Input: part model. Units: mm. Frame: model coordinates. A direction names the side the tool comes from. Coordinates: 2 decimals unless noted, no trailing zeros. Write each loop counter-clockwise with the first axis right and the second up, starting at its lowest first coordinate (ties: lowest second). Pieces come first, ordered by that corner, then holes. Notation, with made-up numbers: (50.5, 17.25) - (79.5, 17.25) arc R13 cw to (79.5, 39.25) - close; hole circle Ø6 at (43.5, 15). An arc over 180 degrees is marked (long way). Put each result on its own line as item: value. Start each with the question number.
1. Cut plane B-B, the plane z = -44. Return loops of the section in (x, y), and give its area (3 significant figures).
2. Access query for faces 1 (the flat face through (5.151, 45.99, -111.247)), 2 (the cylindrical face through (6.28, 102.887, -89.304)), 3 (the flat face through (5, 58.8, -29.4)), 4 (the flat face through (5, -5, -84.398)), 5 (the flat face through (5, -10.16, -117)). Directions: +Z, -Z, +X, -X, +Y, -Y. A direction counts if a zero-diameter tool reaches every point of the face in a straight line with its end or side. Return the directions, or none.
3. Line query: line 1 (Z direction, x = 5.75, y = 66.5); line 2 (Z direction, x = 9, y = 44); line 3 (Y direction, x = 0.5, z = -44). Output: solid intervals per line, ascending.
4. Cut plane A-A, the plane y = 24.5. Return loops of the section in (x, z), and give its area (3 significant figures).
5. Cut plane C-C, the plane z = -133.5. Return loops of the section in (x, y), and give its area (3 significant figures).
6. Pull-direction query (Y, two-part tool) for faces 6 (the flat face through (2.667, -5, -117)), 7 (the flat face through (5.151, 45.99, -38.753)), 8 (the flat face through (5, -10.16, -75)), 9 (the cylindrical face through (2.576, 103.424, -84.174)); classes: released by +Y, released by -Y, zero draft, split by the parting line, or undercut.
7. Pin query (flat end, axial travel): pin 1 (2.5 mm diameter, centred on x = 6, y = -3, fed in from +Z); pin 2 (4 mm diameter, centred on x = 4, y = -3, fed in from -Z); pin 3 (3 mm diameter, centred on x = 6, y = 27, fed in from +Z); pin 4 (5 mm diameter, centred on y = 36, z = -132, fed in from -X). Return the tip coordinate at first contact, or that it passes through.
Autodesk Inventor part; units mm, degrees
ref_plane "YZ Plane" through (0, 0, 0) normal (1, 0, 0) x (0, 1, 0)
ref_plane "XZ Plane" through (0, 0, 0) normal (0, 1, 0) x (-1, 0, 0)
ref_plane "XY Plane" through (0, 0, 0) normal (0, 0, 1) x (1, 0, 0)
sketch "Sketch1" plane through (0, 0, 0) normal (1, 0, 0) x (0, 1, 0)
  line L0 (150, -75) -> (0, 0)
  line L1 (150, -75) -> (0, -150)
  line L2 (0, -150) -> (0, 0)
  dimension "d0" = 150
  dimension "d1" = 75
extrude "Extrusion1" add sketch "Sketch1" along normal blind 10.16
sketch "Sketch2" plane through (10.16, 0, 0) normal (1, 0, 0) x (0, 0, -1)
  point P0 (0, 0)
fillet "Fillet1" radius 19.05 1 edges at (5.08, 150, -75)
sketch "Sketch3" plane through (10.16, 0, 0) normal (1, 0, 0) x (0, 0, -1)
  arc A0 (92.0388, 115.9223) -> (57.9612, 115.9223) centre (75, 107.4029) ccw
  circle A1 centre (75, 107.4029) radius 15
  circle A2 centre (75, 107.4029) radius 10
  line L0 (75, 122.4029) -> (75, 117.4029)
  line L1 (75, 97.4029) -> (75, 92.4029)
  line L2 (85.6066, 118.0095) -> (82.0711, 114.474)
  line L3 (67.9289, 100.3318) -> (64.3934, 96.7963)
  point P0 (0, 0)
  dimension "d5" = 30
  dimension "d34" = 20
  dimension "d35" = 45
  dimension "d36" = 45
sketch "Sketch4" plane through (10.16, 0, 0) normal (1, 0, 0) x (0, 0, -1)
  line L0 (22.8055, 14.0945) -> (60.9055, 90.2945)
  line L1 (57.9612, 115.9223) -> (0, 0)
  line L2 (22.8055, 14.0945) -> (60.9055, 14.0945)
  line L3 (60.9055, 14.0945) -> (60.9055, 90.2945)
  line L4 (0, 0) -> (150, 0) construction
  line L5 (0, 0) -> (150, 0) construction
  arc A0 (92.0388, 115.9223) -> (57.9612, 115.9223) centre (75, 107.4029) ccw construction
  line L6 (75, 126.4529) -> (75, 0) construction
  line L7 (127.1945, 14.0945) -> (89.0945, 90.2945)
  line L8 (127.1945, 14.0945) -> (89.0945, 14.0945)
  line L9 (89.0945, 14.0945) -> (89.0945, 90.2945)
  dimension "d8" = 76.2
  dimension "d11" = 14.0945
  dimension "d12" = 14.0945
  dimension "d13" = 14.0945
extrude "Extrusion3" cut sketch "Sketch4" against normal through all
fillet "Fillet2" radius 5 1 edges at (5.08, 14.0945, -127.1945)
fillet "Fillet3" radius 5 2 edges at (5.08, 14.0945, -89.0945) (5.08, 90.2945, -89.0945)
fillet "Fillet4" radius 5 3 edges at (5.08, 14.0945, -60.9055) (5.08, 90.2945, -60.9055) (5.08, 14.0945, -22.8055)
sketch "Sketch6" plane through (0, 0, -150) normal (0, -1, 0) x (1, 0, 0)
  line L0 (10.16, 150) -> (10.16, 0) construction
  line L1 (10.16, 75) -> (0, 75) construction
  line L2 (0, 65) -> (0, 85) construction
  line L3 (7.493, 126.597) -> (2.667, 126.597)
  line L4 (2.667, 126.597) -> (2.667, 107.801)
  line L5 (2.667, 107.801) -> (7.493, 107.801)
  line L6 (7.493, 107.801) -> (7.493, 126.597)
  line L7 (0, 150) -> (0, 0)
  line L8 (0, 150) -> (10.16, 150)
  line L9 (7.493, 84.398) -> (2.667, 84.398)
  line L10 (2.667, 84.398) -> (2.667, 65.602)
  line L11 (2.667, 65.602) -> (7.493, 65.602)
  line L12 (7.493, 65.602) -> (7.493, 84.398)
  line L13 (7.493, 23.403) -> (2.667, 23.403)
  line L14 (2.667, 23.403) -> (2.667, 42.199)
  line L15 (2.667, 42.199) -> (7.493, 42.199)
  line L16 (7.493, 42.199) -> (7.493, 23.403)
  dimension "d22" = 4.826
  dimension "d23" = 2.667
  dimension "d24" = 2.667
  dimension "d25" = 18.796
  dimension "d26" = 23.403
  dimension "d27" = 18.796
  dimension "d29" = 4.826
  dimension "d30" = 2.667
  dimension "d31" = 2.667
  dimension "d41" = 23.403
extrude "Extrusion5" add sketch "Sketch6" along normal blind 10.16
extrude "Extrusion6" cut sketch "Sketch3" against normal through all contours L2 A2 L0 A1 | A1 L3 A2 L1 | A2
extrude "Extrusion7" cut sketch "Sketch3" against normal blind 5.08 contours A1 L1 A2 L2 | L0 A2 L3 A1
equation "\"d11\" = d13"
equation "\"d12\" = d11"
equation "\"d23\" = d24"
equation "\"d26\" = d41"
equation "\"d27\" = d25"
equation "\"d29\" = d22"
equation "\"d30\" = d23"
properties part number "spool holder arm" material "PLA"
Report:
1. outline: (0, 0) - (10.16, 0) - (10.16, 14.09) - (0, 14.09) - close; (0, 56.48) - (10.16, 56.48) - (10.16, 88) - (0, 88) - close
1. area: 463 mm^2
2. face 1: +X, -X
2. face 2: +X
2. face 3: +Z, +X, -X, +Y
2. face 4: +X, -X, -Y
2. face 5: +Z, -Z, +X, -X, -Y
3. line 1: z = -116.75 to -100.99, -89.09 to -60.91, -49.01 to -33.25
3. line 2: z = -128 to -112.24, -89.09 to -60.91, -37.76 to -22
3. line 3: y = 0 to 14.09, 56.48 to 88
4. outline: (0, -137.75) - (10.16, -137.75) - (10.16, -121.99) - (0, -121.99) - close; (0, -89.09) - (10.16, -89.09) - (10.16, -60.91) - (0, -60.91) - close; (0, -28.01) - (10.16, -28.01) - (10.16, -12.25) - (0, -12.25) - close
4. area: 607 mm^2
5. outline: (0, 0) - (10.16, 0) - (10.16, 33) - (0, 33) - close
5. area: 335 mm^2
6. face 6: zero draft
6. face 7: undercut
6. face 8: released by -Y
6. face 9: undercut
7. pin 1: stops at z = -23.4
7. pin 2: stops at z = -126.6
7. pin 3: stops at z = -12.75
7. pin 4: stops at x = 0
